Autodesk Inventor part; units mm, degrees
ref_plane "YZ Plane" through (0, 0, 0) normal (1, 0, 0) x (0, 1, 0)
ref_plane "XZ Plane" through (0, 0, 0) normal (0, 1, 0) x (-1, 0, 0)
ref_plane "XY Plane" through (0, 0, 0) normal (0, 0, 1) x (1, 0, 0)
sketch "Sketch1" plane through (0, 0, 0) normal (0, 0, 1) x (1, 0, 0)
  line L0 (0, 0) -> (1200, 0)
  line L1 (1200, 0) -> (1200, 16)
  line L2 (1200, 16) -> (0, 16)
  line L3 (0, 16) -> (0, 0)
  dimension "d0" = 1200
  dimension "d1" = 16
extrude "Extrusion1" add sketch "Sketch1" along normal blind 100
sketch "Sketch2" plane through (0, 16, 0) normal (0, 1, 0) x (1, 0, 0)
  line L0 (1200, 0) -> (0, 0)
  line L1 (0, 0) -> (0, -100)
  line L2 (1200, -100) -> (0, -100)
  line L3 (1200, 0) -> (1200, -100)
  line L4 (0, 0) -> (0, -100)
  line L5 (1200, 0) -> (0, 0)
  line L6 (0, 0) -> (0, -16)
  line L7 (0, -16) -> (1200, -16)
  line L8 (1200, -16) -> (1200, 0)
  dimension "d4" = 16
extrude "Extrusion2" add sketch "Sketch2" along normal blind 80 contours L3 L7 L1 L0
properties part number "repisa"
CAD build for the part. Positions are in the model's coordinates, mm. A direction names the side the tool comes from. Round coordinates to 2 decimals unless told otherwise and drop trailing zeros. Order: outer loops, then holes, each group sorted by start corner. A loop starts at its lowest first (then second) coordinate and runs counter-clockwise, first axis right, second up. Notation, with made-up numbers: (3, 70.25) - (35, 70.25) arc R25 ccw to (35, 91.25) - close; hole circle Ø9 at (76, -6). An arc over 180 degrees is marked (long way). Return JSON: item names as keys, results as strings.
(1) Cut at B-B (z = 38). Give the cut face in (x, y), then the cut area to 3 significant figures.
Answer key:
{"outline": "(0, 0) - (1200, 0) - (1200, 16) - (0, 16) - close", "area": "19,200 mm^2"}
(2) Tool access for faces 1 (the face through (608, 16, 57)), 2 (the face through (1200, 15, 27)): list every direction of +Z, -Z, +X, -X, +Y, -Y with a clear straight run to the whole face (end or side of a thin tool).
Answer key:
{"face 1": "+Z, +X, -X, +Y", "face 2": "+Z, -Z, +X, +Y, -Y"}
(3) Cut at A-A (x = 605). Give the cut face in (y, z), then the cut area to 3 significant figures.
Answer key:
{"outline": "(0, 0) - (96, 0) - (96, 16) - (16, 16) - (16, 100) - (0, 100) - close", "area": "2,880 mm^2"}
(4) Wall check: probe 1 along Y at (x, z) = (1084, 59). Give the ranges that are in metal, low to high. Write a range as from..to.
Answer key:
{"probe 1": "y = 0..16"}
(5) Pin check, flat tips, straight feed: pin 1 Ø8 at (x, z) = (965, 73) entering from +Y; pin 2 Ø8 at (x, y) = (524.5, 76.5) entering from +Z. Stop position of each tip, or through.
Answer key:
{"pin 1": "stops at y = 16", "pin 2": "stops at z = 16"}
